Autodesk Inventor part; units mm, degrees
ref_plane "YZ Plane" through (0, 0, 0) normal (1, 0, 0) x (0, 1, 0)
ref_plane "XZ Plane" through (0, 0, 0) normal (0, 1, 0) x (-1, 0, 0)
ref_plane "XY Plane" through (0, 0, 0) normal (0, 0, 1) x (1, 0, 0)
sketch "Sketch1" plane through (0, 0, 0) normal (0, 0, 1) x (1, 0, 0)
  line L0 (0, 0) -> (0, 5.2) construction
  arc A0 (15.6034, 1.2322) -> (-15.6034, 1.2322) centre (0, 5.2) ccw construction
  line L1 (0, 0) -> (0, -5.2) construction
  arc A1 (-15.6034, -1.2322) -> (15.6034, -1.2322) centre (0, -5.2) ccw construction
  line L2 (0, 5.2) -> (0, -5.2) construction
  line L3 (-20.7, 5.2) -> (-20.7, -5.2)
  line L4 (20.7, -5.2) -> (20.7, 5.2)
  arc A2 (20.7, 5.2) -> (-20.7, 5.2) centre (0, 5.2) ccw
  arc A3 (-20.7, -5.2) -> (20.7, -5.2) centre (0, -5.2) ccw
  arc A4 (-15.6034, -1.2322) -> (-15.6034, 1.2322) centre (-20.4492, 0) ccw construction
  arc A5 (15.6034, 1.2322) -> (15.6034, -1.2322) centre (20.4492, 0) ccw construction
  line L5 (0, 5.2) -> (0, -5.2) construction
  circle A6 centre (0, 0) radius 14.5 construction
  dimension "d0" = 10.4
  dimension "d1" = 16.1
  dimension "d2" = 4.6
  dimension "d3" = 5
  dimension "d4" = 41.4
  dimension "d8" = 29
extrude "Extrusion1" add sketch "Sketch1" along normal blind 4
sketch "Sketch2" plane through (0, 0, 4) normal (0, 0, 1) x (1, 0, 0)
  line L0 (-20.7, 5.2) -> (-20.7, -5.2) construction
  arc A0 (-20.7, -5.2) -> (20.7, -5.2) centre (0, -5.2) ccw construction
  line L1 (20.7, -5.2) -> (20.7, 5.2) construction
  arc A1 (20.7, 5.2) -> (-20.7, 5.2) centre (0, 5.2) ccw construction
  line L2 (-18.4, 5.2) -> (-18.4, -5.2) construction
  arc A2 (-18.4, -5.2) -> (18.4, -5.2) centre (0, -5.2) ccw construction
  line L3 (18.4, -5.2) -> (18.4, 5.2) construction
  arc A3 (18.4, 5.2) -> (-18.4, 5.2) centre (0, 5.2) ccw construction
  circle A4 centre (-18.4, 0) radius 1.25
  circle A5 centre (0, 23.6) radius 1.25
  circle A6 centre (-10.6895, 20.1765) radius 1.25
  circle A7 centre (-17.4012, 11.1798) radius 1.25
  line L4 (-18.4, 0) -> (-17.4012, 11.1798) construction
  line L5 (-17.4012, 11.1798) -> (-10.6895, 20.1765) construction
  line L6 (-10.6895, 20.1765) -> (0, 23.6) construction
  line L7 (-18.4, 0) -> (0, 0) construction
  line L8 (0, 0) -> (0, 23.6) construction
  circle A8 centre (18.4, 0) radius 1.25
  circle A9 centre (10.6895, 20.1765) radius 1.25
  circle A10 centre (17.4012, 11.1798) radius 1.25
  circle A11 centre (0, -23.6) radius 1.25
  circle A12 centre (-10.6895, -20.1765) radius 1.25
  circle A13 centre (-17.4012, -11.1798) radius 1.25
  circle A14 centre (10.6895, -20.1765) radius 1.25
  circle A15 centre (17.4012, -11.1798) radius 1.25
  line L9 (-18.4, 0) -> (-18.4, -6) construction
  line L10 (-18.4, -6) -> (-18.628, -6) construction
  line L11 (18.4, 0) -> (18.4, 6) construction
  line L12 (18.4, 6) -> (18.628, 6) construction
  circle A16 centre (-18.628, -6) radius 0.5
  circle A17 centre (18.628, 6) radius 0.5
  dimension "d37" = 2.3
  dimension "d38" = 2.5
  dimension "d39" = 6
  dimension "d40" = 0.228
  dimension "d41" = 6
  dimension "d42" = 0.228
  dimension "d43" = 1
extrude "Extrusion2" cut sketch "Sketch2" against normal through all contours A4 | A5 | A6 | A7 | A8 | A9 | A11 | A12 | A14 | A15 | A16 | A17
sketch "Sketch5" plane through (0, 0, 4) normal (0, 0, 1) x (1, 0, 0)
  line L0 (20.7, -5.2) -> (20.7, 5.2) construction
  arc A0 (20.7, 5.2) -> (-20.7, 5.2) centre (0, 5.2) ccw construction
  line L1 (-20.7, 5.2) -> (-20.7, -5.2) construction
  arc A1 (-20.7, -5.2) -> (20.7, -5.2) centre (0, -5.2) ccw construction
  arc A2 (17.15, 5.2) -> (-17.15, 5.2) centre (0, 5.2) ccw
  line L2 (17.15, 5.2) -> (17.15, -5.2)
  arc A3 (-17.15, -5.2) -> (17.15, -5.2) centre (0, -5.2) ccw
  line L3 (-17.15, -5.2) -> (-17.15, 5.2)
  arc A4 (16.15, 5.2) -> (-16.15, 5.2) centre (0, 5.2) ccw
  line L4 (16.15, 5.2) -> (16.15, -5.2)
  arc A5 (-16.15, -5.2) -> (16.15, -5.2) centre (0, -5.2) ccw
  line L5 (-16.15, -5.2) -> (-16.15, 5.2)
  point P0 (0, 0)
  dimension "d20" = 1
extrude "Extrusion5" cut sketch "Sketch5" against normal blind 0.7
fillet "Fillet1" [suppressed]
chamfer "Chamfer1" distance 1 angle 45 4 edges at (0, -25.9, 0) (20.7, 0, 0) (0, 25.9, 0) (-20.7, 0, 0)
sketch "Sketch8" plane through (0, 0, 0) normal (1, 0, 0) x (0, 1, 0)
  line L0 (0, 0) -> (5.2, 0) construction
  line L1 (0, 0) -> (0, 0.9) construction
  line L2 (-5.2, 4) -> (5.2, 4) construction
  line L3 (0, 4) -> (4.075, 4)
  line L4 (4.075, 4) -> (4.075, 1.4)
  line L5 (4.075, 1.4) -> (3.575, 0.9)
  line L6 (3.575, 0.9) -> (0, 0.9)
  line L7 (0, 0.9) -> (0, 4)
  dimension "d44" = 4.075
  dimension "d45" = 135
  dimension "d46" = 2.6
  dimension "d47" = 0.5
  dimension "d48" = 0.9
revolve "Revolution1" cut sketch "Sketch8" angle 360 about axis through (0, 0, 0.9) along (0, 0, 1)
sketch "Sketch9" plane through (0, 0, 0) normal (0, 0, -1) x (-1, 0, 0)
  circle A0 centre (-18.628, 6) radius 0.5
  circle A1 centre (18.628, -6) radius 0.5
  point P0 (0, 0)
extrude "Extrusion8" add sketch "Sketch9" against normal blind 0.8
properties part number "housingPlate"
Here's how the part is built. I have some questions about the finished solid (model axes, mm). A direction names the side the tool comes from. Coordinates: 2 decimals unless noted, no trailing zeros. Answer in a Markdown table with one row per item.
(1) Will these pins go through, and if not, where does the flat tip stop? pin 1 Ø1.5 at (y, z) = (20.5, 1.5) entering from -X; pin 2 Ø2 at (x, y) = (-10.69, -20.18) entering from +Z; pin 3 Ø1.5 at (x, z) = (7.5, 3.5) entering from -Y.
Answer key:
| item | result |
|---|---|
| pin 1 | x = -14.72 |
| pin 2 | through |
| pin 3 | y = -24.77 |
(2) I want a section at A-A on x = -10.5. Count the separate pieces of the cut face and the enclosed holes in it, then the cut area to 3 significant figures.
Answer key:
| item | result |
|---|---|
| separate pieces | 3 |
| enclosed holes | 0 |
| area | 162 mm^2 |
(3) Thinking about a two-plate mould opening in Y: for faces 1 (the face through (0.672, 24.654, 2.028)), 2 (the face through (-17.56, 12.42, 2.03)), 3 (the face through (0, 5, 4)), which applies, +Y half, -Y half, draft (parallel to the pull), parting line (faces both ways), or undercut?
Answer key:
| item | result |
|---|---|
| face 1 | undercut |
| face 2 | undercut |
| face 3 | draft |
(4) On a 3-axis mill with a long thin cutter (end or side, diameter ignored), from which of +Z, -Z, +X, -X, +Y, -Y can I reach the whole of each face in a straight line? I mean faces 4 (the face through (20.2, -0.1, 0.5)), 5 (the face through (-18.6, -6, 0.8)). Say none if no direction works.
Answer key:
| item | result |
|---|---|
| face 4 | -Z, +X, +Y, -Y |
| face 5 | +Z |
(5) Please list where these lines run through material, in increasing order: probe 1 along Y at (x, z) = (0, 1.5) (3 decimals); probe 2 along X at (y, z) = (1.5, 3.4); probe 3 along X at (y, z) = (10.5, 1.6).
Answer key:
| item | result |
|---|---|
| probe 1 | -25.9 to -24.85, -22.35 to -4.075, 4.075 to 22.35, 24.85 to 25.9 |
| probe 2 | -20.7 to -17.15, -16.15 to -3.79, 3.79 to 16.15, 17.15 to 20.7 |
| probe 3 | -20.01 to -18.45, -16.35 to 20.01 |
